```python
from build123d import *

# Parameters (mm, degrees)
PAD_DEPTH    = 10
SKETCH001_R  = 2.1
POCKET_DEPTH = 5


with BuildPart() as part:
    # Sketch → Pad (new body, symmetric)
    with BuildSketch(Plane.XY):
        Polygon((-5, 4), (-2.5, 4), (-2.5, 4.5), (2.5, 4.5), (2.5, 4), (5, 4), (5, 2.5), (2.5, 0), (-2.5, 0), (-5, 2.5), align=None)
    extrude(amount=PAD_DEPTH, both=True)

    # Sketch001 → Pocket (cut)
    with BuildSketch(Plane.XZ):
        Circle(SKETCH001_R)
    extrude(amount=-POCKET_DEPTH, mode=Mode.SUBTRACT)


solid = part.part
```
The model under review builds one solid part; all positions refer to its coordinate system, in mm. A direction names the side the tool comes from. Coordinates: 2 decimals unless noted, no trailing zeros. Write each loop counter-clockwise with the first axis right and the second up, starting at its lowest first coordinate (ties: lowest second). Pieces come first, ordered by that corner, then holes. Notation, with made-up numbers: (-0.5, 84) - (7.5, 84) arc R17 ccw to (7.5, 97) - close; hole circle Ø1 at (-34, 66.5). An arc over 180 degrees is marked (long way). Answer in a Markdown table with one row per item. Add a question column.
Q1. For faces 4 (the face through (4, 4, 0)), 5 (the face through (-5, 3, 0)), 6 (the face through (-4, 4, 0)), list the 3-axis set-ups (+Z, -Z, +X, -X, +Y, -Y) from which the entire face can be reached by the end or side of a thin tool; tool diameter is ignored.
Q2. To check wall thickness, follow line 1 along Z through (x, y) = (0, 1.15); line 2 along Z through (x, y) = (0.75, 1.2); line 3 along X through (y, z) = (0.35, -8.75). State the ranges of each line that lie inside material, in increasing order. Write a range as from..to.
Q3. Consider section D-D on z = -8.25. Give the boundary of the cut face in (x, y).
Q4. Clearance check with flat-ended pins moving along their axes: pin 1 (0.8 mm diameter, centred on x = -4.5, z = -1.5, fed in from +Y); pin 2 (4 mm diameter, centred on x = 0, z = 0, fed in from -Y). State where each tip first meets the part, or that it passes through.
Q5. Draft analysis for pull direction Z (two halves, no side actions). For faces 1 (the face through (2.003, 2.218, 0.631)), 2 (the face through (0, 2, -10)), 3 (the face through (5, 3, 0)), state which applies: +Z half, -Z half, draft (parallel to the pull), parting line (faces both ways), or undercut.
Q6. Consider section A-A on z = 0. Give the boundary of the cut face in (x, y).
Q7. Consider section C-C on y = 3.4. Give the boundary of the cut face in (x, z).
Q8. Consider section B-B on x = 0. Give the boundary of the cut face in (y, z).
Answers below:
| question | item | result |
|---|---|---|
| 1 | face 4 | +Z, -Z, +X, +Y |
| 1 | face 5 | +Z, -Z, -X, +Y, -Y |
| 1 | face 6 | +Z, -Z, -X, +Y |
| 2 | line 1 | -10..-2.1, 2.1..10 |
| 2 | line 2 | -10..-1.96, 1.96..10 |
| 2 | line 3 | -2.85..2.85 |
| 3 | outline | (-5, 2.5) - (-2.5, 0) - (2.5, 0) - (5, 2.5) - (5, 4) - (2.5, 4) - (2.5, 4.5) - (-2.5, 4.5) - (-2.5, 4) - (-5, 4) - close |
| 4 | pin 1 | y = 4 |
| 4 | pin 2 | through |
| 5 | face 1 | undercut |
| 5 | face 2 | -Z half |
| 5 | face 3 | draft |
| 6 | outline | (-5, 2.5) - (-2.5, 0) - (-2.1, 0) - (-2.1, 4.5) - (-2.5, 4.5) - (-2.5, 4) - (-5, 4) - close; (2.1, 0) - (2.5, 0) - (5, 2.5) - (5, 4) - (2.5, 4) - (2.5, 4.5) - (2.1, 4.5) - close |
| 7 | outline | (-5, -10) - (5, -10) - (5, 10) - (-5, 10) - close; hole circle Ø4.2 at (0, 0) |
| 8 | outline | (0, -10) - (4.5, -10) - (4.5, -2.1) - (0, -2.1) - close; (0, 2.1) - (4.5, 2.1) - (4.5, 10) - (0, 10) - close |
